Could you check a few things on this drawing? It's one solid part, dimensions in mm from its lowest x, y, z. A direction names the side the tool comes from. Give positions to 0.01 mm unless a question says otherwise; leave off trailing zeros. Order: outer loops, then holes, each group sorted by start corner. A loop starts at its lowest first (then second) coordinate and runs counter-clockwise, first axis right, second up. Notation, with made-up numbers: M -33,72 L -21,72 A25 cw -21,97 Z; hole C -8.75,-20 d9. An arc over 180 degrees is marked long. Use one line per item in the form item = value. Start each with the question number.
1. We'd pull the mould along X, two halves only. Please class the marked faces 1 and 2: +X half, -X half, draft (parallel to the pull), parting line (faces both ways), or undercut.
2. I need wall thicknesses on L1, parallel to X at y = 25, z = 0.85; L2, parallel to X at y = 23, z = 4.15; L3, parallel to Y at x = 48, z = 4.8. Which ranges of each line are inside material? Lowest first, please.
3. I want a section at B-B, the plane x = 4.5. List the corners of the cut face in (y, z) for me, and give its area (3 significant figures).
4. For the marked faces 3, 4, 5 and 6, which set-ups out of +Z, -Z, +X, -X, +Y, -Y let a thin tool reach every point of the face, with its end or its side?
5. I want a section at D-D, the plane y = 5. List the corners of the cut face in (x, z) for me.
6. I want a section at A-A, the plane y = 28. List the corners of the cut face in (x, z) for me, and give its area (3 significant figures).
7. I want a section at C-C, the plane z = 1.25. List the corners of the cut face in (x, y) for me.
8. Will these pins go through, and if not, where does the flat tip stop? P1, Ø1.6, axis at y = 20, z = 3, coming from the -X side; P2, Ø1.6, axis at x = 51, z = 2, coming from the -Y side; P3, Ø1.6, axis at x = 49.5, z = 2, coming from the +Y side.
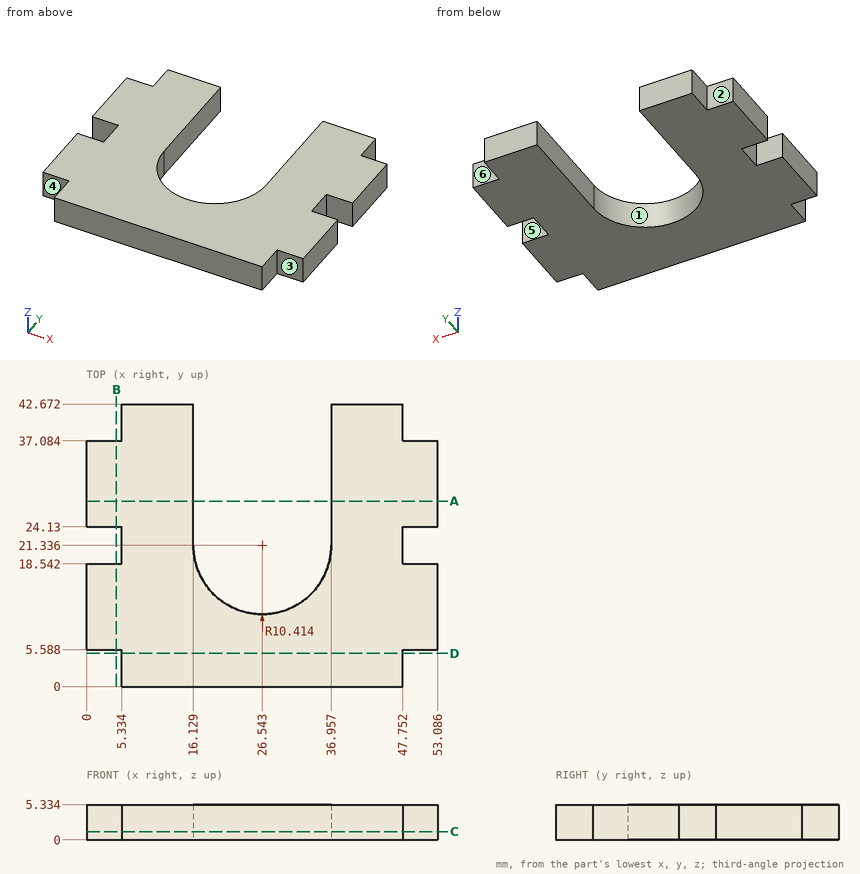
Check result:
q1.face_1 = undercut
q1.face_2 = draft
q2.L1 = 0 to 16.13, 36.96 to 53.09
q2.L2 = 5.33 to 16.13, 36.96 to 47.75
q2.L3 = 5.59 to 18.54, 24.13 to 37.08
q3.outline = M 5.59,0 L 18.54,0 L 18.54,5.33 L 5.59,5.33 Z; M 24.13,0 L 37.08,0 L 37.08,5.33 L 24.13,5.33 Z
q3.area = 138 mm2
q4.face_3 = +Z, -Z, +X, -Y
q4.face_4 = +Z, -Z, -X, -Y
q4.face_5 = +Z, -Z, +X
q4.face_6 = +Z, -Z, +X, +Y
q5.outline = M 5.33,0 L 47.75,0 L 47.75,5.33 L 5.33,5.33 Z
q6.outline = M 0,0 L 16.13,0 L 16.13,5.33 L 0,5.33 Z; M 36.96,0 L 53.09,0 L 53.09,5.33 L 36.96,5.33 Z
q6.area = 172 mm2
q7.outline = M 0,5.59 L 5.33,5.59 L 5.33,0 L 47.75,0 L 47.75,5.59 L 53.09,5.59 L 53.09,18.54 L 47.75,18.54 L 47.75,24.13 L 53.09,24.13 L 53.09,37.08 L 47.75,37.08 L 47.75,42.67 L 36.96,42.67 L 36.96,21.34 A10.41 cw 16.13,21.34 L 16.13,42.67 L 5.33,42.67 L 5.33,37.08 L 0,37.08 L 0,24.13 L 5.33,24.13 L 5.33,18.54 L 0,18.54 Z
q8.P1 = 5.33
q8.P2 = 5.59
q8.P3 = 37.08
